Build history of the part. All positions in model axes, mm. A direction names the side the tool comes from. Give positions to 0.01 mm unless a question says otherwise; leave off trailing zeros. Write each loop counter-clockwise with the first axis right and the second up, starting at its lowest first coordinate (ties: lowest second). Pieces come first, ordered by that corner, then holes. Notation, with made-up numbers: (-24, 46.5) -> (33, 46.5) arc R29 ccw to (33, 66.5) -> close; hole circle Ø2 at (2.25, 37). An arc over 180 degrees is marked (long way). Write item = value, one per line. Start each with the question number.
Q1. Saw through at C-C, the plane y = -9. List the corners of the cut face in (x, z), then the cut area to 3 significant figures.
Q2. Saw through at D-D, the plane x = -12. List the corners of the cut face in (y, z), then the cut area to 3 significant figures.
Q3. Drop flat-ended pins along their axis: P1, Ø14.5, axis at y = -12, z = 53.5, coming from the +X side; P2, Ø6, axis at x = 2, z = 121.5, coming from the -Y side (3 decimals); P3, Ø1, axis at x = 13, z = 21, coming from the +Y side; P4, Ø16.5, axis at x = 7, y = -12.5, coming from the +Z side. Give the stop position or say it passes through.
Q4. Saw through at A-A, the plane x = 12. List the corners of the cut face in (y, z).
Q5. Tool access for faces 1 (the face through (10, -3, 76)), 2 (the face through (-3, 10, 60)), 3 (the face through (-11, -12, 5)): list every direction of +Z, -Z, +X, -X, +Y, -Y with a clear straight run to the whole face (end or side of a thin tool).
Q6. Saw through at B-B, the plane z = 31. List the corners of the cut face in (x, y), then the cut area to 3 significant figures.
Q7. Wall check: line 1 (Y direction, x = -12, z = 1.65); line 2 (X direction, y = 15, z = 4); line 3 (Y direction, x = 6, z = 122). Give the ranges that are in metal, low to high.
Q8. Mould opens along Y. For faces 4 (the face through (10, 3, 76)), 5 (the face through (11.642, 18.227, 2.465)), 6 (the face through (10, 12, 5)) say: pulls with the +Y half, pulls with the -Y half, needs draft (parallel to the pull), parting line crosses it, or undercut.
from build123d import *

# Parameters (mm, degrees)
F0_W     = 15
F0_H     = 18
F0_R     = 2.75
F1_DEPTH = 5
F0_W_2   = 6
F0_H_2   = 6
F2_DEPTH = 150
F3_SIZE2 = 140
F3_SIZE  = 15
F4_SIZE2 = 15
F4_SIZE  = 140
F5_SIZE2 = 12
F5_SIZE  = 140


with BuildPart() as f1:
    # F0 (on Top) → F1 (new body)
    with BuildSketch(Plane.XY):
        with Locations((10.5, 12)):
            Rectangle(F0_W, F0_H)
        with Locations((12, 15.5)):
            Circle(F0_R, mode=Mode.SUBTRACT)
    extrude(amount=F1_DEPTH)



with BuildPart() as f1b:
    # F0 (on Top) → F1, piece 2 (new body)
    with BuildSketch(Plane.XY):
        with Locations((-10.5, 12)):
            Rectangle(F0_W, F0_H)
        with Locations((-12, 15.5)):
            Circle(F0_R, mode=Mode.SUBTRACT)
    extrude(amount=F1_DEPTH)


with BuildPart() as f1c:
    # F0 (on Top) → F1, piece 3 (new body)
    with BuildSketch(Plane.XY):
        with Locations((-10.5, -12)):
            Rectangle(F0_W, F0_H)
        with Locations((-12, -15.5)):
            Circle(F0_R, mode=Mode.SUBTRACT)
    extrude(amount=F1_DEPTH)


with BuildPart() as f1d:
    # F0 (on Top) → F1, piece 4 (new body)
    with BuildSketch(Plane.XY):
        with Locations((10.5, -12)):
            Rectangle(F0_W, F0_H)
        with Locations((12, -15.5)):
            Circle(F0_R, mode=Mode.SUBTRACT)
    extrude(amount=F1_DEPTH)


with BuildPart() as f1_1:
    add(f1.part)

    add(f1b.part)  # F2 merges F1b

    add(f1c.part)  # F2 merges F1c

    add(f1d.part)  # F2 merges F1d
    # F0 (on Top) → F2 (join)
    with BuildSketch(Plane.XY):
        with Locations((0, 12)):
            Rectangle(F0_W_2, F0_H)
        with Locations((0, -12)):
            Rectangle(F0_W_2, F0_H)
        with Locations((10.5, 0)):
            Rectangle(F0_W, F0_H_2)
        with Locations((-10.5, 0)):
            Rectangle(F0_W, F0_H_2)
        Rectangle(F0_W_2, F0_H_2)
    extrude(amount=F2_DEPTH)

    # F3
    f3_edges = [f1_1.edges().sort_by_distance(p)[0] for p in [
        (0, 21, 150),
    ]]
    f3_side = f1_1.faces().sort_by_distance((0, 0, 150))[0]
    chamfer(f3_edges, length=F3_SIZE, length2=F3_SIZE2, reference=f3_side)

    # F4
    f4_edges = [f1_1.edges().sort_by_distance(p)[0] for p in [
        (0, -21, 150),
    ]]
    f4_side = f1_1.faces().sort_by_distance((0, -21, 64.642857))[0]
    chamfer(f4_edges, length=F4_SIZE, length2=F4_SIZE2, reference=f4_side)

    # F5
    f5_edges = [f1_1.edges().sort_by_distance(p)[0] for p in [
        (-18, 0, 150),
    ]]
    f5_side = f1_1.faces().sort_by_distance((-18, 0, 62.916667))[0]
    chamfer(f5_edges, length=F5_SIZE, length2=F5_SIZE2, reference=f5_side)


solid = f1_1.part
Report:
q1.outline = (-18, 0) -> (18, 0) -> (18, 5) -> (3, 5) -> (3, 122) -> (-3, 122) -> (-3, 5) -> (-18, 5) -> close
q1.area = 882 mm2
q2.outline = (-21, 0) -> (-18.25, 0) -> (-18.25, 5) -> (-21, 5) -> close; (-12.75, 0) -> (12.75, 0) -> (12.75, 5) -> (3, 5) -> (3, 80) -> (-3, 80) -> (-3, 5) -> (-12.75, 5) -> close; (18.25, 0) -> (21, 0) -> (21, 5) -> (18.25, 5) -> close
q2.area = 605 mm2
q3.P1 = 3
q3.P2 = -9.375
q3.P3 = 3
q3.P4 = 150
q4.outline = (-21, 0) -> (-18.25, 0) -> (-18.25, 5) -> (-21, 5) -> close; (-12.75, 0) -> (12.75, 0) -> (12.75, 5) -> (3, 5) -> (3, 150) -> (-3, 150) -> (-3, 5) -> (-12.75, 5) -> close; (18.25, 0) -> (21, 0) -> (21, 5) -> (18.25, 5) -> close
q5.face_1 = +Z, +X, -Y
q5.face_2 = +Z, -X, +Y
q5.face_3 = +Z, -X, -Y
q6.outline = (-16.2, -3) -> (-3, -3) -> (-3, -18.75) -> (3, -18.75) -> (3, -3) -> (18, -3) -> (18, 3) -> (3, 3) -> (3, 18.75) -> (-3, 18.75) -> (-3, 3) -> (-16.2, 3) -> close
q6.area = 394 mm2
q7.line_1 = -21 to -18.25, -12.75 to 12.75, 18.25 to 21
q7.line_2 = -18 to -14.7, -9.3 to 9.3, 14.7 to 18
q7.line_3 = -3 to 3
q8.face_4 = pulls with the +Y half
q8.face_5 = undercut
q8.face_6 = needs draft
